Geometry check sheet. Reference: the model listing, model coordinates, mm. Face numbers are marked on the shaded views. A direction names the side the tool comes from. Coordinates: 2 decimals unless noted, no trailing zeros. Order: outer loops, then holes, each group sorted by start corner. A loop starts at its lowest first (then second) coordinate and runs counter-clockwise, first axis right, second up. Notation, with made-up numbers: (37, 34.25) - (69, 34.25) arc R20 cw to (69, 58.25) - close; hole circle Ø8 at (64.5, 32). An arc over 180 degrees is marked (long way). Use CSV: the item, a comma, the result in double quotes. Start each with the question number.
1) Draft check along X on the marked faces 1, 2, 3 and 4. Enter one of: released by +X, released by -X, zero draft, split by the parting line, or undercut.
2) Sectioned sample at B-B, the plane y = 6. Record the cut outline in (x, z).
3) Depth check by flat-ended pin: P1, Ø5, axis at y = 43, z = 10, coming from the -X side; P2, Ø8, axis at x = -20, y = 26.5, coming from the +Z side; P3, Ø1.8, axis at y = 43, z = -10, coming from the +X side. Enter the tip coordinate at first touch or a pass-through.
4) Thickness scan on probe 1 along Y at (x, z) = (-28, 27); probe 2 along Z at (x, y) = (8, 26). Record the ranges inside material, lowest first. Write a range as [from, to].
5) Sectioned sample at A-A, the plane x = 35. Record the cut outline in (y, z), and give its area (3 significant figures).
6) Sectioned sample at D-D, the plane y = 35.5. Record the cut outline in (x, z).
7) Tool access check on the marked faces 5, 6 and 7. Record the directions out of +Z, -Z, +X, -X, +Y, -Y that give a thin tool (end or side, any length) a straight path to the whole face; none if there is none.
8) Sectioned sample at C-C, the plane x = 0. Record the cut outline in (y, z), and give its area (3 significant figures).
from build123d import *

# Parameters (mm, degrees)
SKETCH1_W           = 100
SKETCH1_H           = 60
BOSS_EXTRUDE2_DEPTH = 20
SKETCH2_R           = 15
SKETCH2_R_2         = 10
BOSS_EXTRUDE3_DEPTH = 30
SKETCH3_W           = 14
SKETCH3_H           = 35.201995264
CUT_EXTRUDE1_DEPTH  = 10
RIB4_REACH          = 78.811
SKETCH19_WALL_W     = 186.230224572
SKETCH19_WALL_H     = 6


with BuildPart() as part:
    # Sketch1 → Boss-Extrude2 (new body)
    with BuildSketch(Plane(origin=(0, 0, 0), x_dir=(1, 0, 0), z_dir=(0, 1, 0))):
        Rectangle(SKETCH1_W, SKETCH1_H)
        with BuildLine():
            ThreePointArc((-44.951219512, -10), (-35, -19.951219512), (-25.048780488, -10))
            Line((-25.048780488, -10), (-25.048780488, 10))
            ThreePointArc((-25.048780488, 10), (-35, 19.951219512), (-44.951219512, 10))
            Line((-44.951219512, 10), (-44.951219512, -10))
        make_face(mode=Mode.SUBTRACT)
        with BuildLine():
            Line((44.951219512, 10), (44.951219512, -10))
            ThreePointArc((44.951219512, -10), (35, -19.951219512), (25.048780488, -10))
            Line((25.048780488, -10), (25.048780488, 10))
            ThreePointArc((25.048780488, 10), (35, 19.951219512), (44.951219512, 10))
        make_face(mode=Mode.SUBTRACT)
        with BuildLine():
            Line((-44.951219512, 10), (-44.951219512, -10))
            ThreePointArc((-44.951219512, -10), (-35, -19.951219512), (-25.048780488, -10))
            Line((-25.048780488, -10), (-25.048780488, 10))
            ThreePointArc((-25.048780488, 10), (-35, 19.951219512), (-44.951219512, 10))
        make_face()
        with BuildLine():
            ThreePointArc((-40.268292683, -10), (-35, -15.268292683), (-29.731707317, -10))
            Line((-29.731707317, -10), (-29.731707317, 10))
            ThreePointArc((-29.731707317, 10), (-35, 15.268292683), (-40.268292683, 10))
            Line((-40.268292683, 10), (-40.268292683, -10))
        make_face(mode=Mode.SUBTRACT)
        with BuildLine():
            ThreePointArc((44.951219512, -10), (35, -19.951219512), (25.048780488, -10))
            Line((25.048780488, -10), (25.048780488, 10))
            ThreePointArc((25.048780488, 10), (35, 19.951219512), (44.951219512, 10))
            Line((44.951219512, 10), (44.951219512, -10))
        make_face()
        with BuildLine():
            Line((40.268292683, 10), (40.268292683, -10))
            ThreePointArc((40.268292683, -10), (35, -15.268292683), (29.731707317, -10))
            Line((29.731707317, -10), (29.731707317, 10))
            ThreePointArc((29.731707317, 10), (35, 15.268292683), (40.268292683, 10))
        make_face(mode=Mode.SUBTRACT)
    extrude(amount=BOSS_EXTRUDE2_DEPTH)

    # Sketch2 → Boss-Extrude3 (add)
    with BuildSketch(Plane(origin=(0, 20, 0), x_dir=(1, 0, 0), z_dir=(0, 1, 0))):
        with Locations(Location((0, 0, 0), (0, 0, 270))):
            Circle(SKETCH2_R)
        with Locations(Location((0, 0, 0), (0, 0, 270))):
            Circle(SKETCH2_R_2, mode=Mode.SUBTRACT)
    extrude(amount=BOSS_EXTRUDE3_DEPTH)

    # Sketch3 → Cut-Extrude1 (cut)
    with BuildSketch(Plane(origin=(0, 50, 0), x_dir=(1, 0, 0), z_dir=(0, 1, 0))):
        Rectangle(SKETCH3_W, SKETCH3_H)
    extrude(amount=-CUT_EXTRUDE1_DEPTH, mode=Mode.SUBTRACT)

    # Sketch19 wall → Rib4 (add, up to next)
    with BuildSketch(Plane(origin=(20, 34.463811754, 0), x_dir=(0.32671934012, -0.945121406377, 0), z_dir=(0.945121406377, 0.32671934012, 0)), mode=Mode.PRIVATE) as rib4_sk1:
        Rectangle(SKETCH19_WALL_W, SKETCH19_WALL_H)
    rib4_tool1 = extrude(rib4_sk1.sketch, amount=-RIB4_REACH, mode=Mode.PRIVATE) - part.part
    rib4 = rib4_tool1.solids().sort_by_distance((20, 34.463811754, 0))[0]
    add(rib4)

    # Mirror2: Rib4 across plane
    add(rib4.mirror(Plane(origin=(0, 0, 0), x_dir=(0, 0, 1), z_dir=(1, 0, 0))))


solid = part.part
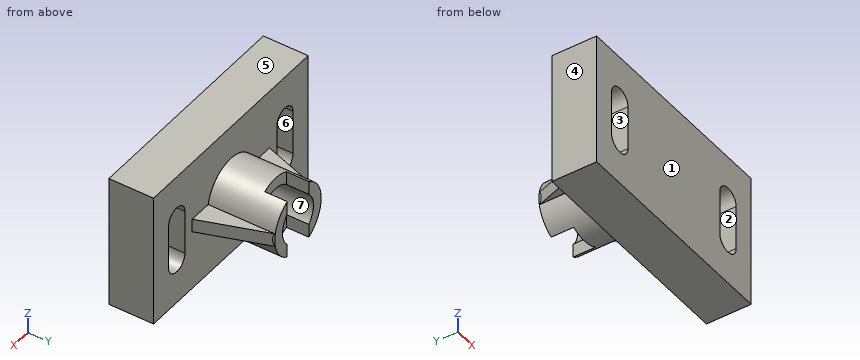
Evaluation:
1,face 1,"zero draft"
1,face 2,"undercut"
1,face 3,"undercut"
1,face 4,"released by -X"
2,outline,"(-50, -30) - (50, -30) - (50, 30) - (-50, 30) - close; hole (-40.27, -10) arc R5.27 ccw to (-29.73, -10) - (-29.73, 10) arc R5.27 ccw to (-40.27, 10) - close; hole (29.73, -10) arc R5.27 ccw to (40.27, -10) - (40.27, 10) arc R5.27 ccw to (29.73, 10) - close"
3,P1,"x = -12.99"
3,P2,"z = 3"
3,P3,"x = 11.92"
4,probe 1,"[0, 20]"
4,probe 2,"[-12.69, -6], [6, 12.69]"
5,outline,"(0, -30) - (20, -30) - (20, -15.27) - (0, -15.27) - close; (0, 15.27) - (20, 15.27) - (20, 30) - (0, 30) - close"
5,area,"589 mm²"
6,outline,"(-19.64, -3) - (-14.7, -3) arc R15 ccw to (14.7, -3) - (19.64, -3) - (19.64, 3) - (14.7, 3) arc R15 ccw to (-14.7, 3) - (-19.64, 3) - close; hole circle Ø20 at (0, 0)"
7,face 5,"+Z, +X, -X, +Y, -Y"
7,face 6,"+Y, -Y"
7,face 7,"+Y"
8,outline,"(0, -30) - (20, -30) - (20, -15) - (40, -15) - (40, -10) - (20, -10) - (20, 10) - (40, 10) - (40, 15) - (20, 15) - (20, 30) - (0, 30) - close"
8,area,"1,400 mm²"
